Verification items for the finished model (mm, model axes). Face numbers are marked on the shaded views. A direction names the side the tool comes from. Coordinates: 2 decimals unless noted, no trailing zeros. Write each loop counter-clockwise with the first axis right and the second up, starting at its lowest first coordinate (ties: lowest second). Pieces come first, ordered by that corner, then holes. Notation, with made-up numbers: (24.5, -28.5) -> (46.5, -28.5) arc R20 cw to (46.5, -17.5) -> close; hole circle Ø9 at (45.25, 15). An arc over 180 degrees is marked (long way). Write each question's results on one line, items separated by ' | '. Start each with the question number.
from build123d import *

# Parameters (mm, degrees)
SKETCH1_W                    = 3.175
SKETCH1_H                    = 30
BASE_FLANGE1_DEPTH           = 15
EDGE_FLANGE1_STRIP_W         = 14.1732
EDGE_FLANGE1_STRIP_H         = 3.175
EDGE_FLANGE1_STRIP_CUT_DEPTH = 30
EDGE_FLANGE1_DEPTH           = 30


# Sheet-metal steps are written as plain solids
with BuildPart() as part:
    # Sketch1 → Base-Flange1 (new body)
    with BuildSketch(Plane(origin=(0, 0, 0), x_dir=(0, 0, -1), z_dir=(1, 0, 0))):
        with Locations((1.5875, 0)):
            Rectangle(SKETCH1_W, SKETCH1_H)
    extrude(amount=BASE_FLANGE1_DEPTH)

    # Edge-Flange1 strip (across the edge) → Edge-Flange1 strip cut (cut)
    with BuildSketch(Plane.XZ.offset(-15)):
        with Locations((-3.175, -1.5875)):
            Rectangle(EDGE_FLANGE1_STRIP_W, EDGE_FLANGE1_STRIP_H)
    extrude(amount=EDGE_FLANGE1_STRIP_CUT_DEPTH, mode=Mode.SUBTRACT)

    # Edge-Flange1 section (across the edge) → Edge-Flange1 (add)
    with BuildSketch(Plane.XZ.offset(-15)):
        with BuildLine():
            Line((0, 0.7366), (0, 11.825))
            Line((0, 11.825), (3.175, 11.825))
            Line((3.175, 11.825), (3.175, 0.7366))
            ThreePointArc((3.175, 0.7366), (3.390745145, 0.215745145), (3.9116, 0))
            Line((3.9116, 0), (3.9116, -3.175))
            ThreePointArc((3.9116, -3.175), (1.145681115, -2.029318885), (0, 0.7366))
        make_face()
    extrude(amount=EDGE_FLANGE1_DEPTH)


solid = part.part
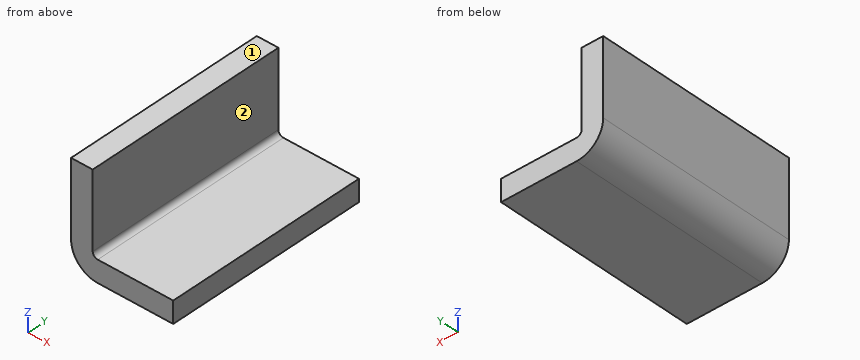
1. Material ranges on probe 1 along X at (y, z) = (-11, 3) (3 decimals); probe 2 along Z at (x, y) = (7, 8.5) (3 decimals); probe 3 along Z at (x, y) = (2.5, 1.5) (3 decimals), recorded low to high. Write a range as from..to.
2. Sectioned sample at A-A on y = 5.25. Record the cut outline in (x, z) (3 decimals).
3. Tool access check on the marked faces 1 and 2. Record the directions out of +Z, -Z, +X, -X, +Y, -Y that give a thin tool (end or side, any length) a straight path to the whole face; none if there is none.
4. Sectioned sample at C-C on z = 10. Record the cut outline in (x, y) (3 decimals).
5. Sectioned sample at B-B on x = 7.5. Record the cut outline in (y, z) (3 decimals), plus the area to 4 significant figures.
6. Depth check by flat-ended pin: pin 1 Ø5.5 at (y, z) = (4.5, 5) entering from +X (3 decimals); pin 2 Ø1 at (x, y) = (10.5, 9) entering from +Z; pin 3 Ø5 at (x, z) = (10.5, 4) entering from +Y. Enter the tip coordinate at first touch or a pass-through.
Computed values:
1) probe 1: x = 0..3.175 | probe 2: z = -3.175..0 | probe 3: z = -2.911..11.825
2) outline: (0, 0.737) arc R3.912 ccw to (3.912, -3.175) -> (15, -3.175) -> (15, 0) -> (3.912, 0) arc R0.737 cw to (3.175, 0.737) -> (3.175, 11.825) -> (0, 11.825) -> close
3) face 1: +Z, +X, -X, +Y, -Y | face 2: +Z, +X, +Y, -Y
4) outline: (0, -15) -> (3.175, -15) -> (3.175, 15) -> (0, 15) -> close
5) outline: (-15, -3.175) -> (15, -3.175) -> (15, 0) -> (-15, 0) -> close | area: 95.25 mm^2
6) pin 1: stops at x = 3.175 | pin 2: stops at z = 0 | pin 3: passes through
